Geometry: final body of the model. Coordinates: model frame, mm. Coordinates: 2 decimals unless noted, no trailing zeros. Write each loop counter-clockwise with the first axis right and the second up, starting at its lowest first coordinate (ties: lowest second). Pieces come first, ordered by that corner, then holes. Notation, with made-up numbers: (16.5, 31) - (68.5, 31) arc R19 ccw to (68.5, 59) - close; hole circle Ø7 at (-35.75, -12.5). An arc over 180 degrees is marked (long way). Answer as a JSON object with one key per item and string values. Group by question number.
Item 1: Section C-C on x = 19.05. Return loops of the section in (y, z), and give its area (3 significant figures).
Item 2: Line query: line 1 along Z through (x, y) = (19.5, 1.1); line 2 along Z through (x, y) = (19, -0.8); line 3 along X through (y, z) = (-0.5, 17.5). Output: solid intervals per line, ascending. Write a range as from..to.
Item 3: Section A-A on y = 0.8. State how many separate pieces and enclosed holes the cut face has, and give its area (3 significant figures).
Item 4: Section B-B on z = 0. Return loops of the section in (x, y).
Item 5: Section D-D on z = 15. Return loops of the section in (x, y).
Item 6: First-contact query: pin 1 Ø4 at (x, z) = (-20, 0) entering from -Y; pin 2 Ø6 at (x, z) = (20, 15.5) entering from +Y. Flat tips, straight axial feed; report the tip coordinate or a pass-through.
Item 7: Mould query, pull axis X, two halves, no side actions, for faces 1 (the flat face through (16.813, 0.022, 14.633)), 2 (the flat face through (0, 1.588, 0)), 3 (the cylindrical face through (-21.16, -0.02, -1.1)). Classes: pulls with the +X half, pulls with the -X half, needs draft (parallel to the pull), parting line crosses it, or undercut.
```python
from build123d import *

# Parameters (mm, degrees)
BOSS_EXTRUDE1_DEPTH            = 1.5875
F_3_16_0_1875_DIAMETER_HOLE1_D = 4.7625


with BuildPart() as part:
    # Sketch1 → Boss-Extrude1 (new, symmetric)
    with BuildSketch(Plane(origin=(0, 0, 0), x_dir=(1, 0, 0), z_dir=(0, 1, 0))):
        with BuildLine():
            Line((24.308582085, 3.559468282), (9.525, 25.4))
            Line((9.525, 25.4), (-9.525, 25.4))
            Line((-9.525, 25.4), (-24.308582085, 3.559468282))
            ThreePointArc((-24.308582085, 3.559468282), (-25.4, 0), (-24.308582085, -3.559468282))
            Line((-24.308582085, -3.559468282), (-9.525, -25.4))
            Line((-9.525, -25.4), (9.525, -25.4))
            Line((9.525, -25.4), (24.308582085, -3.559468282))
            ThreePointArc((24.308582085, -3.559468282), (25.4, 0), (24.308582085, 3.559468282))
        make_face()
    extrude(amount=BOSS_EXTRUDE1_DEPTH, both=True)

    # 3/16 (0.1875) Diameter Hole1 (through all)
    with Locations(Plane(origin=(19.05, 1.5875, 0), x_dir=(0, 0, 1), z_dir=(0, 1, 0))):
        with Locations((0, 0), (0, -38.1)):
            Hole(F_3_16_0_1875_DIAMETER_HOLE1_D / 2)


solid = part.part
```
Checks:
{
 "1": {"outline": "(-1.59, -11.33) - (1.59, -11.33) - (1.59, -2.38) - (-1.59, -2.38) - close; (-1.59, 2.38) - (1.59, 2.38) - (1.59, 11.33) - (-1.59, 11.33) - close", "area": "56.8 mm^2"},
 "2": {"line 1": "-10.66..-2.34, 2.34..10.66", "line 2": "-11.4..-2.38, 2.38..11.4", "line 3": "-14.87..14.87"},
 "3": {"separate pieces": "1", "enclosed holes": "2", "area": "1,800 mm^2"},
 "4": {"outline": "(-25.4, -1.59) - (-21.43, -1.59) - (-21.43, 1.59) - (-25.4, 1.59) - close; (-16.67, -1.59) - (16.67, -1.59) - (16.67, 1.59) - (-16.67, 1.59) - close; (21.43, -1.59) - (25.4, -1.59) - (25.4, 1.59) - (21.43, 1.59) - close"},
 "5": {"outline": "(-16.56, -1.59) - (16.56, -1.59) - (16.56, 1.59) - (-16.56, 1.59) - close"},
 "6": {"pin 1": "y = -1.59", "pin 2": "through"},
 "7": {"face 1": "pulls with the +X half", "face 2": "needs draft", "face 3": "undercut"}
}
